Answer from the drawing. Dimensions are ordinates in mm from the lowest x, y and z of the part. A direction names the side the tool comes from. Coordinates: 2 decimals unless noted, no trailing zeros. Order: outer loops, then holes, each group sorted by start corner. A loop starts at its lowest first (then second) coordinate and runs counter-clockwise, first axis right, second up. Notation, with made-up numbers: (22.25, 87) - (30.25, 87) arc R20 cw to (30.25, 110) - close; hole circle Ø11 at (-7.75, -7.75). An arc over 180 degrees is marked (long way). Answer as a JSON object with one key per item and string values. Group by question number.
1) Section D-D (z = 40.64) is taken. Give the vertices of the cut face in (x, y), plus the area to 3 significant figures.
2) A tool of negligible diameter and unlimited length cuts with its end or side. For the marked faces 1 and 2, from which of +Z, -Z, +X, -X, +Y, -Y can it reach the whole face along a straight path? Write none if from no direction.
3) Find the intervals of material crossed by line 1 along X through (y, z) = (3, 40.64); line 2 along Y through (x, z) = (25.4, 2.75) (1 decimal); line 3 along Z through (x, y) = (40.64, 8), in increasing order.
4) Section B-B (x = 25.4) is taken. Count the separate pieces of the cut face and the enclosed holes in it.
5) Each of these flat-tipped pins is pushed along its axis until it touches: P1, Ø3, axis at x = 25.5, y = 6.5, coming from the -Z side; P2, Ø8, axis at x = 20, z = 21, coming from the +Y side; P3, Ø12, axis at x = 36.5, y = 38.5, coming from the +Z side. Where does it stop, or does it pass through?
6) Section C-C (y = 14) is taken. Give the vertices of the cut face in (x, z).
7) Section A-A (z = 22) is taken. Give the vertices of the cut face in (x, y) (1 decimal).
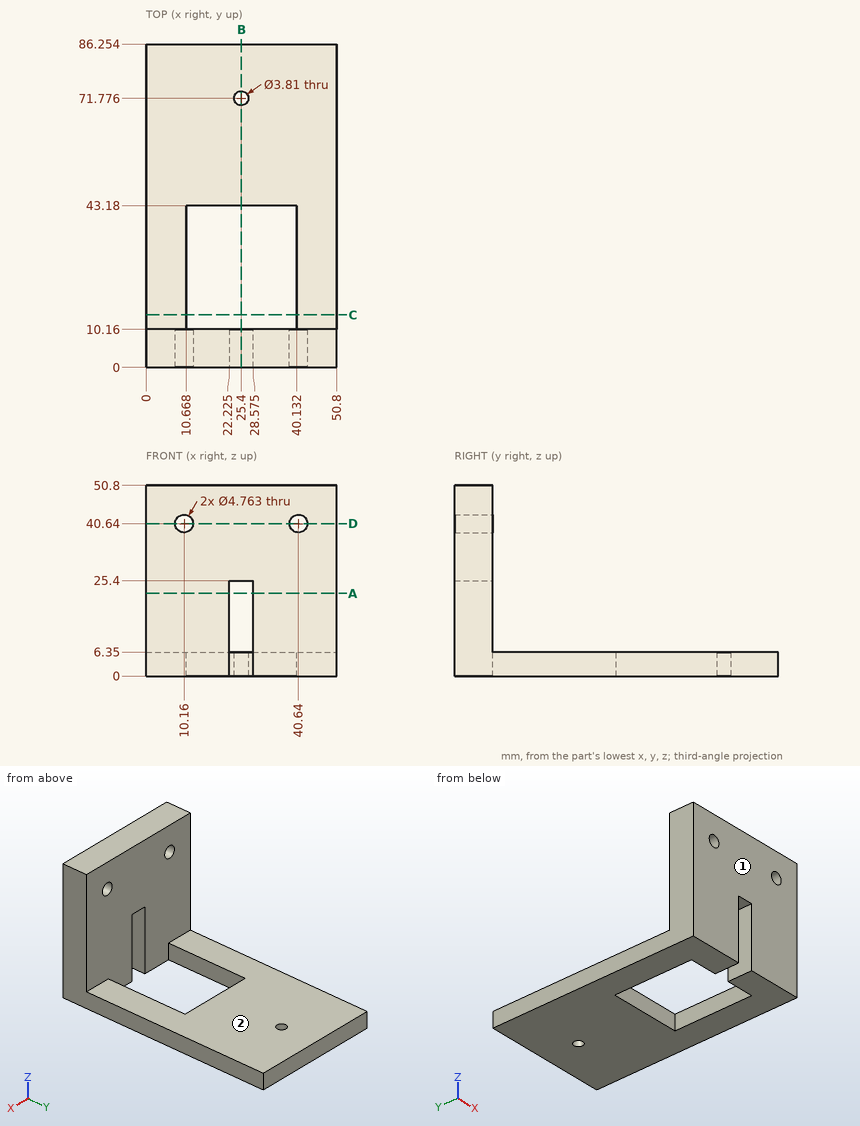
Report:
{
 "1": {"outline": "(0, 0) - (7.78, 0) - (7.78, 10.16) - (0, 10.16) - close; (12.54, 0) - (38.26, 0) - (38.26, 10.16) - (12.54, 10.16) - close; (43.02, 0) - (50.8, 0) - (50.8, 10.16) - (43.02, 10.16) - close", "area": "419 mm²"},
 "2": {"face 1": "+Z, -Z, +X, -X, -Y", "face 2": "+Z, +X, -X, +Y"},
 "3": {"line 1": "x = 0 to 7.78, 12.54 to 38.26, 43.02 to 50.8", "line 2": "y = 43.2 to 69.9, 73.7 to 86.3", "line 3": "z = 0 to 38.26, 43.02 to 50.8"},
 "4": {"separate pieces": "3", "enclosed holes": "0"},
 "5": {"P1": "stops at z = 25.4", "P2": "stops at y = 10.16", "P3": "stops at z = 6.35"},
 "6": {"outline": "(0, 0) - (10.67, 0) - (10.67, 6.35) - (0, 6.35) - close; (40.13, 0) - (50.8, 0) - (50.8, 6.35) - (40.13, 6.35) - close"},
 "7": {"outline": "(0, 0) - (22.2, 0) - (22.2, 10.2) - (0, 10.2) - close; (28.6, 0) - (50.8, 0) - (50.8, 10.2) - (28.6, 10.2) - close"}
}
